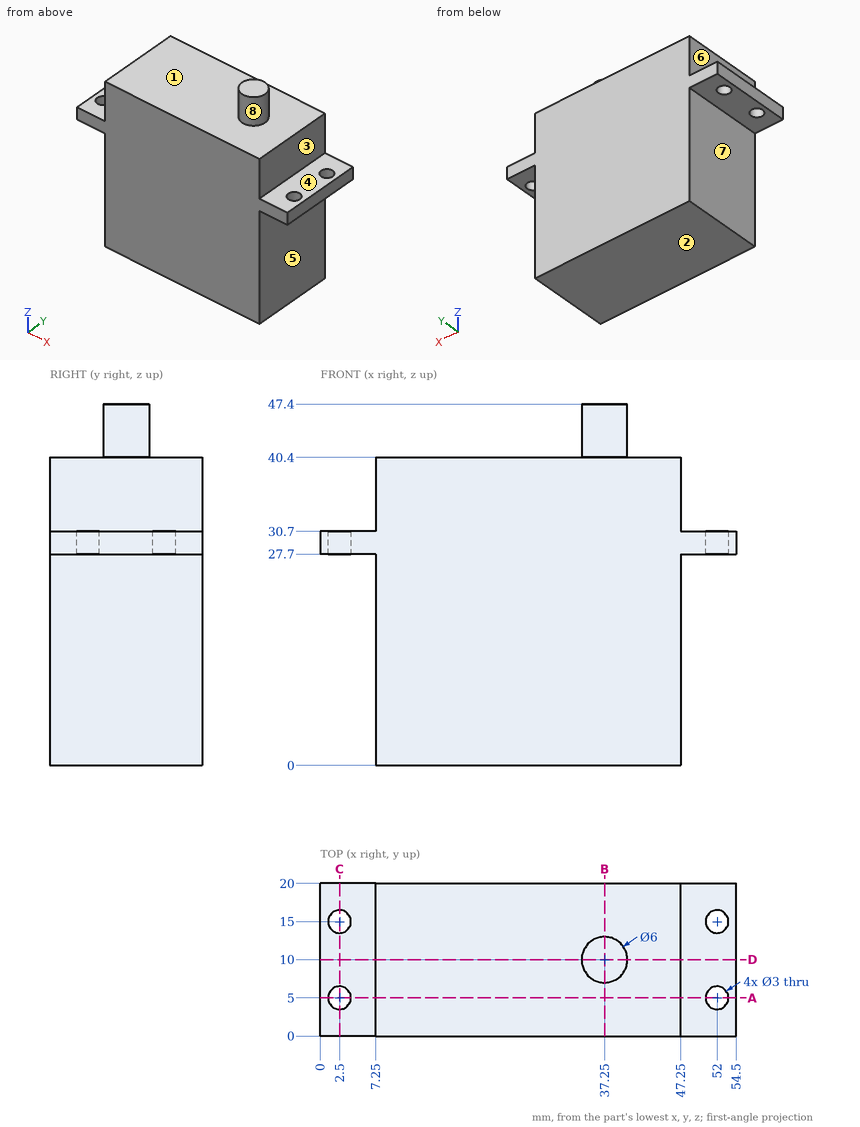
Verification items for this drawing (mm, ordinates from the low corner). A direction names the side the tool comes from. Coordinates: 2 decimals unless noted, no trailing zeros. Order: outer loops, then holes, each group sorted by start corner. A loop starts at its lowest first (then second) coordinate and runs counter-clockwise, first axis right, second up. Notation, with made-up numbers: (6, 6.25) -> (23, 6.25) arc R28 ccw to (23, 44.25) -> close; hole circle Ø5 at (26, 41). An arc over 180 degrees is marked (long way). Answer as CSV lines item,"result". Start each with the question number.
1) Cross-section at A-A, the plane y = 5. Record the boundary of the cut face in (x, z).
2) Cross-section at B-B, the plane x = 37.25. Record the boundary of the cut face in (y, z), then the cut area to 3 significant figures.
3) Cross-section at C-C, the plane x = 2.5. Record the boundary of the cut face in (y, z).
4) Material ranges on L1, parallel to Y at x = 2.5, z = 29.2; L2, parallel to Z at x = 43.5, y = 18.75; L3, parallel to X at y = 13, z = 18, recorded low to high. Write a range as [from, to].
5) Cross-section at D-D, the plane y = 10. Record the boundary of the cut face in (x, z), then the cut area to 3 significant figures.
6) Release check for a two-part mould opening along Z. For the marked faces 1, 2 and 3 record: released by +Z, released by -Z, zero draft, split by the parting line, or undercut.
7) Gauge pin test, flat ends, axial feed: pin 1 Ø6 at (y, z) = (9.5, 37) entering from +X; pin 2 Ø3.5 at (x, y) = (51, 15) entering from -Z; pin 3 Ø2 at (y, z) = (4, 41.5) entering from +X; pin 4 Ø6 at (x, y) = (50, 12) entering from +Z. Record the tip position at first contact, or that the pin passes through.
8) Set-up check for the marked faces 4, 5, 6, 7 and 8: record each of +Z, -Z, +X, -X, +Y, -Y from which the full face is reachable in a straight line by a thin tool's end or side.
Conclusion:
1,outline,"(0, 27.7) -> (1, 27.7) -> (1, 30.7) -> (0, 30.7) -> close; (4, 27.7) -> (7.25, 27.7) -> (7.25, 0) -> (47.25, 0) -> (47.25, 27.7) -> (50.5, 27.7) -> (50.5, 30.7) -> (47.25, 30.7) -> (47.25, 40.4) -> (7.25, 40.4) -> (7.25, 30.7) -> (4, 30.7) -> close; (53.5, 27.7) -> (54.5, 27.7) -> (54.5, 30.7) -> (53.5, 30.7) -> close"
2,outline,"(0, 0) -> (20, 0) -> (20, 40.4) -> (13, 40.4) -> (13, 47.4) -> (7, 47.4) -> (7, 40.4) -> (0, 40.4) -> close"
2,area,"850 mm²"
3,outline,"(0, 27.7) -> (3.5, 27.7) -> (3.5, 30.7) -> (0, 30.7) -> close; (6.5, 27.7) -> (13.5, 27.7) -> (13.5, 30.7) -> (6.5, 30.7) -> close; (16.5, 27.7) -> (20, 27.7) -> (20, 30.7) -> (16.5, 30.7) -> close"
4,L1,"y = [0, 3.5], [6.5, 13.5], [16.5, 20]"
4,L2,"z = [0, 40.4]"
4,L3,"x = [7.25, 47.25]"
5,outline,"(0, 27.7) -> (7.25, 27.7) -> (7.25, 0) -> (47.25, 0) -> (47.25, 27.7) -> (54.5, 27.7) -> (54.5, 30.7) -> (47.25, 30.7) -> (47.25, 40.4) -> (40.25, 40.4) -> (40.25, 47.4) -> (34.25, 47.4) -> (34.25, 40.4) -> (7.25, 40.4) -> (7.25, 30.7) -> (0, 30.7) -> close"
5,area,"1,700 mm²"
6,face 1,"released by +Z"
6,face 2,"released by -Z"
6,face 3,"zero draft"
7,pin 1,"stops at x = 47.25"
7,pin 2,"stops at z = 27.7"
7,pin 3,"passes through"
7,pin 4,"stops at z = 40.4"
8,face 4,"+Z, +X, +Y, -Y"
8,face 5,"-Z, +X, +Y, -Y"
8,face 6,"+Z, -X, +Y, -Y"
8,face 7,"-Z, -X, +Y, -Y"
8,face 8,"+Z"
